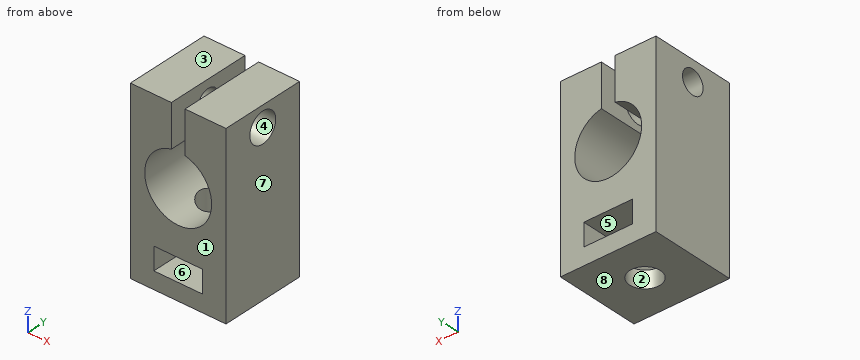
```python
from build123d import *

# Parameters (mm, degrees)
F0_W     = 14
F0_H     = 26
F0_W_2   = 7.15
F0_H_2   = 3.3
F0_R     = 4.9
F1_DEPTH = 12.5
F2_R     = 2.25
F3_DEPTH = 15
F4_W     = 2
F4_H     = 9.3737413222
F5_DEPTH = 12.5010001
F6_R     = 1.75
F7_DEPTH = 14.001
F8_R     = 2.2
F9_DEPTH = 6


with BuildPart() as f1:
    # F0 (on Front) → F1 (new body)
    with BuildSketch(Plane.XZ):
        with Locations((0, -2)):
            Rectangle(F0_W, F0_H)
        with Locations((0, -10.85)):
            Rectangle(F0_W_2, F0_H_2, mode=Mode.SUBTRACT)
        Circle(F0_R, mode=Mode.SUBTRACT)
    extrude(amount=F1_DEPTH)

    # F2 (on face) → F3 (cut)
    with BuildSketch(Plane(origin=(0, 0, -15), x_dir=(1, 0, 0), z_dir=(0, 0, -1))):
        with Locations((0, 6.25)):
            Circle(F2_R)
    extrude(amount=-F3_DEPTH, mode=Mode.SUBTRACT)

    # F4 (on face) → F5 (cut, through all)
    with BuildSketch(Plane.XZ.offset(12.5)):
        with Locations((0, 6.3131293389)):
            Rectangle(F4_W, F4_H)
    extrude(amount=-F5_DEPTH, mode=Mode.SUBTRACT)

    # F6 (on face) → F7 (cut, through all)
    with BuildSketch(Plane.YZ.offset(7)):
        with Locations((-6.25, 8)):
            Circle(F6_R)
    extrude(amount=-F7_DEPTH, mode=Mode.SUBTRACT)

    # F8 (on face) → F9 (cut)
    with BuildSketch(Plane.YZ.offset(7)):
        with Locations((-6.25, 8)):
            Circle(F8_R)
    extrude(amount=-F9_DEPTH, mode=Mode.SUBTRACT)


solid = f1.part
```
The listing builds one solid part. Answer for the finished solid, in the listing's coordinates (mm). Face numbers are marked on the shaded views. A direction names the side the tool comes from. Give positions to 0.01 mm unless a question says otherwise; leave off trailing zeros. Order: outer loops, then holes, each group sorted by start corner. A loop starts at its lowest first (then second) coordinate and runs counter-clockwise, first axis right, second up. Notation, with made-up numbers: (-21.5, 0.25) - (5.5, 0.25) arc R34 cw to (5.5, 34.25) - close; hole circle Ø3 at (25, 34). An arc over 180 degrees is marked (long way). Answer in a Markdown table with one row per item. Add a question column.
Q1. Find the intervals of material crossed by line 1 along X through (y, z) = (-9, 7.75); line 2 along X through (y, z) = (-3.75, 0); line 3 along Y through (x, z) = (0, -7.45), in increasing order. Write a range as [from, to].
Q2. Given P1, Ø2.5, axis at x = 0, y = -6.25, coming from the -Z side, flat-ended and moving along its own axis, determine where the tip first touches the part or whether it passes through.
Q3. Which of the six approach directions +Z, -Z, +X, -X, +Y, -Y give full straight-line access (tool end or side, diameter ignored) to the marked faces 1, 2, 3, 4 and 5?
Q4. The part is cut by section D-D (x = 4.5). Determine the outline of the cut face in (y, z), then the cut area to 3 significant figures.
Q5. The part is cut by section C-C (y = -6.25). Determine the outline of the cut face in (x, z) (3 decimals), then the cut area to 3 significant figures.
Q6. For a pull along Z with two mould halves and no side action, classify the marked faces 6, 7 and 8 as released by +Z, released by -Z, zero draft, split by the parting line, or undercut.
Q7. The part is cut by section B-B (z = 8). Determine the outline of the cut face in (x, y), then the cut area to 3 significant figures.
Q8. The part is cut by section A-A (x = 0). Determine the outline of the cut face in (y, z).
Determined:
| question | item | result |
|---|---|---|
| 1 | line 1 | x = [-7, -1], [1, 7] |
| 1 | line 2 | x = [-7, -4.9], [4.9, 7] |
| 1 | line 3 | y = [-12.5, -8.5], [-4, 0] |
| 2 | P1 | stops at z = 4.74 |
| 3 | face 1 | +Z, -Z, +X, -X, -Y |
| 3 | face 2 | -Z |
| 3 | face 3 | +Z, +X, -X, +Y, -Y |
| 3 | face 4 | +X |
| 3 | face 5 | +Y, -Y |
| 4 | outline | (-12.5, -15) - (0, -15) - (0, -1.94) - (-12.5, -1.94) - close; (-12.5, 1.94) - (0, 1.94) - (0, 11) - (-12.5, 11) - close; hole circle Ø4.4 at (-6.25, 8) |
| 4 | area | 261 mm² |
| 5 | outline | (-7, -15) - (-2.25, -15) - (-2.25, -12.5) - (-3.575, -12.5) - (-3.575, -9.2) - (-2.25, -9.2) - (-2.25, -4.353) arc R4.9 cw to (-1, 4.797) - (-1, 6.25) - (-7, 6.25) - close; (-7, 9.75) - (-1, 9.75) - (-1, 11) - (-7, 11) - close; (1, 4.797) arc R4.9 cw to (2.25, -4.353) - (2.25, -9.2) - (3.575, -9.2) - (3.575, -12.5) - (2.25, -12.5) - (2.25, -15) - (7, -15) - (7, 5.8) - (1, 5.8) - close; (1, 10.2) - (7, 10.2) - (7, 11) - (1, 11) - close |
| 5 | area | 174 mm² |
| 6 | face 6 | undercut |
| 6 | face 7 | zero draft |
| 6 | face 8 | released by -Z |
| 7 | outline | (-7, -12.5) - (-1, -12.5) - (-1, -8) - (-7, -8) - close; (-7, -4.5) - (-1, -4.5) - (-1, 0) - (-7, 0) - close; (1, -12.5) - (7, -12.5) - (7, -8.45) - (1, -8.45) - close; (1, -4.05) - (7, -4.05) - (7, 0) - (1, 0) - close |
| 7 | area | 103 mm² |
| 8 | outline | (-12.5, -15) - (-8.5, -15) - (-8.5, -12.5) - (-12.5, -12.5) - close; (-12.5, -9.2) - (-8.5, -9.2) - (-8.5, -4.9) - (-12.5, -4.9) - close; (-4, -15) - (0, -15) - (0, -12.5) - (-4, -12.5) - close; (-4, -9.2) - (0, -9.2) - (0, -4.9) - (-4, -4.9) - close |
